Can you work these out from the model? Positions are in its coordinate system, mm. Face numbers are marked on the shaded views. A direction names the side the tool comes from. Round coordinates to 2 decimals unless told otherwise and drop trailing zeros. Order: outer loops, then holes, each group sorted by start corner. A loop starts at its lowest first (then second) coordinate and runs counter-clockwise, first axis right, second up. Notation, with made-up numbers: (33.5, -18.75) -> (90.5, -18.75) arc R26 ccw to (90.5, -0.75) -> close; hole circle Ø5 at (78.25, 69). An arc over 180 degrees is marked (long way). Use a Markdown table: item, result. Add a question column.
Q1. We'd pull the mould along Z, two halves only. Please class the marked faces 3, 4, 5 and 6: +Z half, -Z half, draft (parallel to the pull), parting line (faces both ways), or undercut.
Q2. For the marked faces 1 and 2, which set-ups out of +Z, -Z, +X, -X, +Y, -Y let a thin tool reach every point of the face, with its end or its side?
Q3. I'm going to push a flat-ended pin straight in: pin 1 Ø1.5 at (x, z) = (0.5, 0.5) entering from +Y. Where does the tip first touch, or does it pass through?
Q4. I need wall thicknesses on line 1 along Z through (x, y) = (1.35, 14.5); line 2 along X through (y, z) = (5.5, -1.65); line 3 along Z through (x, y) = (1.85, 2). Which ranges of each line are inside material? Lowest first, please. Write a range as [from, to].
Q5. If we section it at C-C on z = 0.65: List the corners of the cut face in (x, y) for me.
Q6. If we section it at A-A on y = 11.5: List the corners of the cut face in (x, z) for me, plus the area to 3 significant figures.
Q7. If we section it at B-B on x = -0.5: List the corners of the cut face in (y, z) for me.
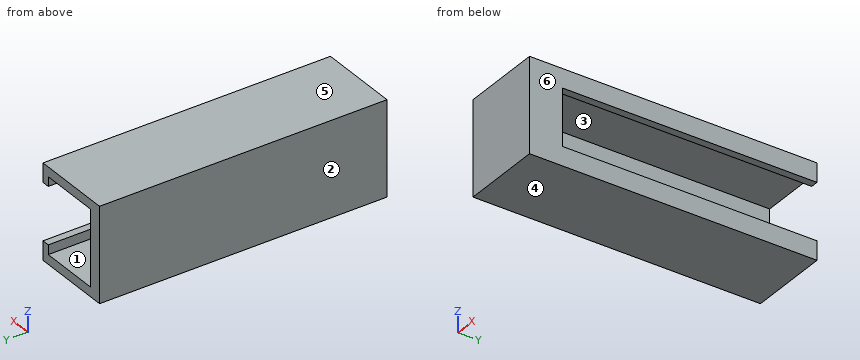
```python
from build123d import *

# Parameters (mm, degrees)
SKETCH1_W           = 4.3
SKETCH1_H           = 15.2
BOSS_EXTRUDE1_DEPTH = 2.5
CUT_EXTRUDE1_START  = -1.75
CUT_EXTRUDE1_DEPTH  = 14.45


with BuildPart() as part:
    # Sketch1 → Boss-Extrude1 (new body, symmetric)
    with BuildSketch(Plane.XY):
        with Locations((0, 7.6)):
            Rectangle(SKETCH1_W, SKETCH1_H)
    extrude(amount=BOSS_EXTRUDE1_DEPTH, both=True)

    # Sketch3 → Cut-Extrude1 (cut, through all)
    with BuildSketch(Plane(origin=(0, 0, 0), x_dir=(-1, 0, 0), z_dir=(0, -1, 0)).offset(CUT_EXTRUDE1_START)):
        Polygon((-2.15, -1.5), (-1.75, -1.5), (-1.75, -2), (1.45, -2), (1.45, 2), (-1.75, 2), (-1.75, 1.5), (-2.15, 1.5), align=None)
    extrude(amount=-CUT_EXTRUDE1_DEPTH, mode=Mode.SUBTRACT)


solid = part.part
```
Answer below:
| question | item | result |
|---|---|---|
| 1 | face 3 | undercut |
| 1 | face 4 | -Z half |
| 1 | face 5 | +Z half |
| 1 | face 6 | draft |
| 2 | face 1 | +Y |
| 2 | face 2 | +Z, -Z, -X, +Y, -Y |
| 3 | pin 1 | y = 1.75 |
| 4 | line 1 | [-2.5, -2], [2, 2.5] |
| 4 | line 2 | [-2.15, -1.45], [1.75, 2.15] |
| 4 | line 3 | [-2.5, -1.5], [1.5, 2.5] |
| 5 | outline | (-2.15, 0) -> (2.15, 0) -> (2.15, 1.75) -> (-1.45, 1.75) -> (-1.45, 15.2) -> (-2.15, 15.2) -> close |
| 6 | outline | (-2.15, -2.5) -> (2.15, -2.5) -> (2.15, -1.5) -> (1.75, -1.5) -> (1.75, -2) -> (-1.45, -2) -> (-1.45, 2) -> (1.75, 2) -> (1.75, 1.5) -> (2.15, 1.5) -> (2.15, 2.5) -> (-2.15, 2.5) -> close |
| 6 | area | 7.50 mm² |
| 7 | outline | (0, -2.5) -> (15.2, -2.5) -> (15.2, -2) -> (1.75, -2) -> (1.75, 2) -> (15.2, 2) -> (15.2, 2.5) -> (0, 2.5) -> close |
